```python
from build123d import *

# Parameters (mm, degrees)
F0_R     = 3
F1_DEPTH = 3


# Not quite as in the source:
# - a feature names something its author has since deleted; it is built from what else it names


with BuildPart() as f1:
    # F0 (on Front) → F1 (new body)
    with BuildSketch(Plane.XZ):
        with BuildLine():
            ThreePointArc((18, -80), (25.2450835608, -57.9435000854), (37.8911830779, -38.474124356))
            ThreePointArc((37.8911830779, -38.474124356), (59.2223421632, -23.3521866114), (84, -15))
            Line((84, -15), (84, 30))
            ThreePointArc((84, 30), (43.0306603199, 43.8097481595), (0, 48))
            ThreePointArc((0, 48), (-43.0306603199, 43.8097481595), (-84, 30))
            Line((-84, 30), (-84, -15))
            ThreePointArc((-84, -15), (-59.2223421632, -23.3521866114), (-37.8911830779, -38.474124356))
            ThreePointArc((-37.8911830779, -38.474124356), (-25.2450835608, -57.9435000854), (-18, -80))
            Line((-18, -80), (0, -80))
            Line((0, -80), (18, -80))
        make_face()
        with Locations((-30.3108891325, -17.5)):
            Circle(F0_R, mode=Mode.SUBTRACT)
        with Locations((0, -35)):
            Circle(F0_R, mode=Mode.SUBTRACT)
        with Locations((30.3108891325, -17.5)):
            Circle(F0_R, mode=Mode.SUBTRACT)
        with Locations((-30.3108891325, 17.5)):
            Circle(F0_R, mode=Mode.SUBTRACT)
        with BuildLine():
            ThreePointArc((19.2964358267, -19.5933040702), (-25.3663358138, 10.6206877076), (27.5, 0))
            ThreePointArc((27.5, 0), (25.3663358138, -10.6206877076), (19.2964358267, -19.5933040702))
        make_face(mode=Mode.SUBTRACT)
        with Locations((30.3108891325, 17.5)):
            Circle(F0_R, mode=Mode.SUBTRACT)
        with Locations((0, 35)):
            Circle(F0_R, mode=Mode.SUBTRACT)
    extrude(amount=F1_DEPTH)


solid = f1.part
```
Verification items for the finished model (mm, model axes). Give positions to 0.01 mm unless a question says otherwise; leave off trailing zeros. Write each loop counter-clockwise with the first axis right and the second up, starting at its lowest first coordinate (ties: lowest second). Pieces come first, ordered by that corner, then holes. Notation, with made-up numbers: (36, 86.25) - (70, 86.25) arc R24 ccw to (70, 114.25) - close; hole circle Ø2 at (35.5, 80.5). An arc over 180 degrees is marked (long way). Put each result on its own line as item: value.
Q1. Section check D-D on z = -17.5. Record the cut outline in (x, y), and give its area (3 significant figures).
Result:
outline: (-73.71, -3) - (-33.31, -3) - (-33.31, 0) - (-73.71, 0) - close; (-27.31, -3) - (-21.21, -3) - (-21.21, 0) - (-27.31, 0) - close; (21.21, -3) - (27.31, -3) - (27.31, 0) - (21.21, 0) - close; (33.31, -3) - (73.71, -3) - (73.71, 0) - (33.31, 0) - close
area: 279 mm2
Q2. Scan lines: probe 1 along X at (y, z) = (-2.05, 15); probe 2 along Z at (x, y) = (4, -2.6); probe 3 along Z at (x, y) = (53, -0.2). Record each from-to range of solid material in increasing order. Write a range as from..to.
Result:
probe 1: -84..-31.97, -28.65..-23.05, 23.05..28.65, 31.97..84
probe 2: -80..-27.21, 27.21..48.03
probe 3: -26.84..41.39
Q3. Section check B-B on z = 5. Record the cut outline in (x, y), and give its area (3 significant figures).
Result:
outline: (-84, -3) - (-27.04, -3) - (-27.04, 0) - (-84, 0) - close; (27.04, -3) - (84, -3) - (84, 0) - (27.04, 0) - close
area: 342 mm2
Q4. Section check C-C on x = 12. Record the cut outline in (y, z).
Result:
outline: (-3, -80) - (0, -80) - (0, -24.74) - (-3, -24.74) - close; (-3, 24.74) - (0, 24.74) - (0, 47.82) - (-3, 47.82) - close
Q5. Depth check by flat-ended pin: P1, Ø7, axis at x = 0, z = 35, coming from the +Y side; P2, Ø5.5, axis at x = 30.31, z = -17.5, coming from the +Y side; P3, Ø1.5, axis at x = 39.5, y = -1, coming from the -Z side. Enter the tip coordinate at first touch or a pass-through.
Result:
P1: y = 0
P2: through
P3: z = -37.66
Q6. Section check A-A on y = -1.1. Record the cut outline in (x, z), and give its area (3 significant figures).
Result:
outline: (-84, -15) arc R90 cw to (-37.89, -38.47) arc R90 cw to (-18, -80) - (18, -80) arc R90 cw to (37.89, -38.47) arc R90 cw to (84, -15) - (84, 30) arc R190 ccw to (0, 48) arc R190 ccw to (-84, 30) - close; hole circle Ø6 at (-30.31, -17.5); hole circle Ø6 at (-30.31, 17.5); hole circle Ø55 at (0, 0); hole circle Ø6 at (0, -35); hole circle Ø6 at (0, 35); hole circle Ø6 at (30.31, -17.5); hole circle Ø6 at (30.31, 17.5)
area: 11,800 mm2
Q7. Mould release check, pull along X, two halves, no side actions. Record for faces 1 (the face through (27.314, -1.479, 17.632)), 2 (the face through (-59.55, -1.479, -23.186)), 3 (the face through (25.105, -1.479, -58.238)): released by +X, released by -X, zero draft, split by the parting line, or undercut.
Result:
face 1: undercut
face 2: released by -X
face 3: released by +X
